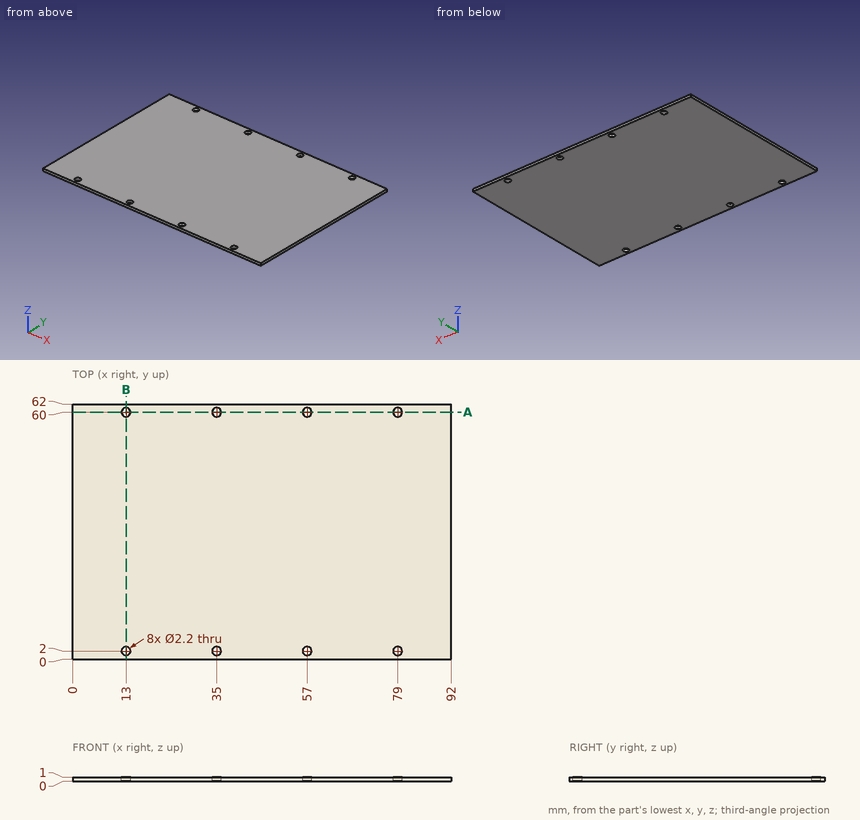
Geometry check sheet. Reference: drawing and pictorial views, mm from the part's lowest x, y, z. Round coordinates to 2 decimals unless told otherwise and drop trailing zeros. Write each loop counter-clockwise with the first axis right and the second up, starting at its lowest first coordinate (ties: lowest second). Pieces come first, ordered by that corner, then holes. Notation, with made-up numbers: (-24, -3.75) -> (16, -3.75) arc R30 ccw to (16, 22.25) -> close; hole circle Ø10 at (-6.5, 52.5). An arc over 180 degrees is marked (long way). Answer as CSV lines item,"result". Start each with the question number.
1) Material ranges on line 1 (Y direction, x = 57, z = 0.4); line 2 (X direction, y = 3, z = 0.1); line 3 (Y direction, x = 56.5, z = 0.1), recorded low to high. Write a range as from..to.
2) Section check A-A on y = 60. Enter the section's corners in (x, z), and give its area (3 significant figures).
3) Section check B-B on x = 13. Enter the section's corners in (y, z).
Found:
1,line 1,"y = 0..0.9, 3.1..58.9, 61.1..62"
1,line 2,"x = 0..12.54, 13.46..34.54, 35.46..56.54, 57.46..78.54, 79.46..92"
1,line 3,"y = 0..1.02, 2.98..59.02, 60.98..62"
2,outline,"(0, 0) -> (11.9, 0) -> (11.9, 1) -> (0, 1) -> close; (14.1, 0) -> (33.9, 0) -> (33.9, 1) -> (14.1, 1) -> close; (36.1, 0) -> (55.9, 0) -> (55.9, 1) -> (36.1, 1) -> close; (58.1, 0) -> (77.9, 0) -> (77.9, 1) -> (58.1, 1) -> close; (80.1, 0) -> (92, 0) -> (92, 1) -> (80.1, 1) -> close"
2,area,"83.2 mm^2"
3,outline,"(0, 0) -> (0.9, 0) -> (0.9, 1) -> (0, 1) -> close; (3.1, 0) -> (58.9, 0) -> (58.9, 1) -> (3.1, 1) -> close; (61.1, 0) -> (62, 0) -> (62, 1) -> (61.1, 1) -> close"
